Source: CAD feature listing. Evaluate the final solid. Frame: model axes, mm. A direction names the side the tool comes from. Round coordinates to 2 decimals unless told otherwise and drop trailing zeros. Write each loop counter-clockwise with the first axis right and the second up, starting at its lowest first coordinate (ties: lowest second). Pieces come first, ordered by that corner, then holes. Notation, with made-up numbers: M -2.75,88.25 L 54.25,88.25 A20 cw 54.25,96.25 Z; hole C 40,55.25 d1. An arc over 180 degrees is marked long. Answer in a Markdown table with one row per item.
from build123d import *

# Parameters (mm, degrees)
CROQUIS1_W              = 100
CROQUIS1_H              = 100
SALIENTE_EXTRUIR1_DEPTH = 20
CROQUIS2_R              = 1.5
CORTAR_EXTRUIR1_DEPTH   = 28
CROQUIS3_W              = 7.071067812
CROQUIS3_H              = 7.071067812
CORTAR_EXTRUIR2_DEPTH   = 18
VACIADO1_START          = -48
VACIADO1_OUTLINE_W      = 18
VACIADO1_OUTLINE_H      = 81.857864376
VACIADO1_DEPTH          = 96
VACIADO1_START_2        = -40.928932188
VACIADO1_2_OUTLINE_W    = 18
VACIADO1_2_OUTLINE_H    = 7.071067812
VACIADO1_2_DEPTH        = 81.857864376


# Read off the part's stored shape, not the designer's step: Vaciado1
with BuildPart() as part:
    # Croquis1 → Saliente-Extruir1 (new body)
    with BuildSketch(Plane(origin=(0, 0, 0), x_dir=(1, 0, 0), z_dir=(0, 1, 0))):
        Rectangle(CROQUIS1_W, CROQUIS1_H)
    extrude(amount=SALIENTE_EXTRUIR1_DEPTH)

    # Croquis2 → Cortar-Extruir1 (cut)
    with BuildSketch(Plane(origin=(0, 20, 0), x_dir=(1, 0, 0), z_dir=(0, 1, 0))):
        with Locations(Location((-46.464466094, -46.464466094, 0), (0, 0, 270))):
            Circle(CROQUIS2_R)
        with Locations(Location((-46.464466094, 46.464466094, 0), (0, 0, 270))):
            Circle(CROQUIS2_R)
        with Locations(Location((46.464466094, 46.464466094, 0), (0, 0, 270))):
            Circle(CROQUIS2_R)
        with Locations(Location((46.464466094, -46.464466094, 0), (0, 0, 270))):
            Circle(CROQUIS2_R)
    extrude(amount=-CORTAR_EXTRUIR1_DEPTH, mode=Mode.SUBTRACT)

    # Croquis3 → Cortar-Extruir2 (cut)
    with BuildSketch(Plane(origin=(0, 20, 0), x_dir=(1, 0, 0), z_dir=(0, 1, 0))):
        with Locations((-46.464466094, -46.464466094)):
            Rectangle(CROQUIS3_W, CROQUIS3_H)
        with Locations((-46.464466094, 46.464466094)):
            Rectangle(CROQUIS3_W, CROQUIS3_H)
        with Locations((46.464466094, 46.464466094)):
            Rectangle(CROQUIS3_W, CROQUIS3_H)
        with Locations((46.464466094, -46.464466094)):
            Rectangle(CROQUIS3_W, CROQUIS3_H)
    extrude(amount=-CORTAR_EXTRUIR2_DEPTH, mode=Mode.SUBTRACT)

    # Vaciado1 outline → Vaciado1 (cut)
    with BuildSketch(Plane.YZ.offset(VACIADO1_START)):
        with Locations((9, 0)):
            Rectangle(VACIADO1_OUTLINE_W, VACIADO1_OUTLINE_H)
    extrude(amount=VACIADO1_DEPTH, mode=Mode.SUBTRACT)

    # Vaciado1 2 outline → Vaciado1 2 (cut)
    with BuildSketch(Plane.YZ.offset(VACIADO1_START_2)):
        with Locations((9, -44.464466094)):
            Rectangle(VACIADO1_2_OUTLINE_W, VACIADO1_2_OUTLINE_H)
        with Locations((9, 44.464466094)):
            Rectangle(VACIADO1_2_OUTLINE_W, VACIADO1_2_OUTLINE_H)
    extrude(amount=VACIADO1_2_DEPTH, mode=Mode.SUBTRACT)


solid = part.part
Q1. Section C-C (z = 18). Return loops of the section in (x, y).
Solutions:
| item | result |
|---|---|
| outline | M -50,0 L -48,0 L -48,18 L 48,18 L 48,0 L 50,0 L 50,20 L -50,20 Z |
Q2. Section B-B (x = 5.5). Return loops of the section in (y, z), and give its area (3 significant figures).
Solutions:
| item | result |
|---|---|
| outline | M 0,-50 L 20,-50 L 20,50 L 0,50 L 0,48 L 18,48 L 18,-48 L 0,-48 Z |
| area | 272 mm2 |
Q3. Section A-A (y = 5). Return loops of the section in (x, z).
Solutions:
| item | result |
|---|---|
| outline | M -50,-42.93 L -42.93,-42.93 L -42.93,-50 L 42.93,-50 L 42.93,-42.93 L 50,-42.93 L 50,42.93 L 42.93,42.93 L 42.93,50 L -42.93,50 L -42.93,42.93 L -50,42.93 Z; hole M -48,-40.93 L -40.93,-40.93 L -40.93,-48 L 40.93,-48 L 40.93,-40.93 L 48,-40.93 L 48,40.93 L 40.93,40.93 L 40.93,48 L -40.93,48 L -40.93,40.93 L -48,40.93 Z |
Q4. Pull-direction query (X, two-part tool) for faces 1 (the flat face through (46, 11, 42.929)), 2 (the flat face through (-50, 10, 1)), 3 (the flat face through (-45, 9, 40.929)); classes: pulls with the +X half, pulls with the -X half, needs draft (parallel to the pull), parting line crosses it, or undercut.
Solutions:
| item | result |
|---|---|
| face 1 | needs draft |
| face 2 | pulls with the -X half |
| face 3 | undercut |
Q5. Material intervals for probe 1 along Z at (x, y) = (-28, 8.5); probe 2 along Z at (x, y) = (41, 3), sorted ascending.
Solutions:
| item | result |
|---|---|
| probe 1 | z = -50 to -48, 48 to 50 |
| probe 2 | z = -50 to -40.93, 40.93 to 50 |
Q6. Contact query for flat-ended pins moving along their axis: pin 1 Ø3 at (x, z) = (-26, 12) entering from -Y; pin 2 Ø2 at (y, z) = (11.5, 44) entering from +X; pin 3 Ø3.5 at (x, y) = (-47, 6.5) entering from -Z. Output: stop coordinate, or through.
Solutions:
| item | result |
|---|---|
| pin 1 | stops at y = 18 |
| pin 2 | stops at x = 42.93 |
| pin 3 | stops at z = -42.93 |
Q7. Access query for faces 4 (the flat face through (-42.929, 11, 47)), 5 (the flat face through (-1, 20, -1)), 6 (the flat face through (-48.1, 2, -47.3)), 7 (the flat face through (-1, 9, -48)). Directions: +Z, -Z, +X, -X, +Y, -Y. A direction counts if a zero-diameter tool reaches every point of the face in a straight line with its end or side. Return the directions, or none.
Solutions:
| item | result |
|---|---|
| face 4 | +Z, -X, +Y |
| face 5 | +Z, -Z, +X, -X, +Y |
| face 6 | -Z, -X, +Y |
| face 7 | -Y |
